Input: part model. Units: mm. Frame: model coordinates. Face numbers are marked on the shaded views. A direction names the side the tool comes from. Round coordinates to 2 decimals unless told otherwise and drop trailing zeros. Loops run counter-clockwise (first coordinate to the right, second up) from the corner with the lowest first, then second, coordinate; pieces in that order, holes last.
1) Ray query, line 1 along X through (y, z) = (8.75, -10); line 2 along Z through (x, y) = (130, 3.25); line 3 along Z through (x, y) = (169, 13.25). Return the intervals inside material, ascending.
2) First-contact query: pin 1 (1.2 mm diameter, centred on x = 75, z = -10, fed in from +Y); pin 2 (1 mm diameter, centred on x = 178, z = 10.5, fed in from -Y); pin 3 (12 mm diameter, centred on x = 121, y = 10.5, fed in from +Z); pin 4 (1.5 mm diameter, centred on y = 9, z = 55.5, fed in from -X). Flat tips, straight axial feed; report the tip coordinate or a pass-through.
3) Access query for the marked faces 1 and 2. Directions: +Z, -Z, +X, -X, +Y, -Y. A direction counts if a zero-diameter tool reaches every point of the face in a straight line with its end or side. Return the directions, or none.
4) Section A-A, the plane z = -114. Return loops of the section in (x, y).
5) Draft query along X for the marked faces 3, 4, 5 and 6. Return one class per face: pulls with the +X half, pulls with the -X half, needs draft (parallel to the pull), parting line crosses it, or undercut.
6) Section B-B, the plane x = 151.5. Return loops of the section in (y, z).
from build123d import *

# Parameters (mm, degrees)
CORNERBOSS_EXTRUDE1_DEPTH               = 20
SHELL1_T                                = -3
PUTBACKPARTOFSHELLBOSS_EXTRUDE1_DEPTH   = 17
TABHOLECUTSSKETCH1_R                    = 1
TABHOLECUTS_EXTRUDE3_DEPTH              = 267.480732183
PADSKETCH2_R                            = 12
PADSKETCH2_R_2                          = 5
PADBOSS_EXTRUDE2_DEPTH                  = 10
STEPPERRODHOLESKETCH3_R                 = 5.1
STEPPERRODHOLESKETCH3_R_2               = 1.5
STEPPERRODHOLECUT_EXTRUDE1_DEPTH        = 267.046951918
THREADEDNUTMOUNTHOLESSKETCH4_R          = 1
THREADEDNUTMOUNTHOLESCUT_EXTRUDE2_DEPTH = 10
TLPEGHOLESKETCH1_W                      = 10
TLPEGHOLESKETCH1_H                      = 14
TLPEGHOLECUT_EXTRUDE1_DEPTH             = 3
BOTTOMPEGSKETCH2_W                      = 9.8
BOTTOMPEGSKETCH2_H                      = 13.9
BOTTOMPEGBOSS_EXTRUDE1_DEPTH            = 3.1
BOTTOMPEGCAPSKETCH3_W                   = 16
BOTTOMPEGCAPSKETCH3_H                   = 17
BOTTOMPEGCAPBOSS_EXTRUDE2_DEPTH         = 3


with BuildPart() as part:
    # CornerSketch1 → CornerBoss-Extrude1 (new body)
    with BuildSketch(Plane(origin=(0, 0, 0), x_dir=(1, 0, 0), z_dir=(0, 1, 0))):
        with BuildLine():
            Line((210, -50), (120, -50))
            Line((120, -50), (120, 0))
            Line((120, 0), (0, 0))
            Line((0, 0), (0, 100))
            Line((0, 100), (176, 100))
            Line((176, 100), (176, 145.825))
            ThreePointArc((176, 145.825), (193, 162.825), (210, 145.825))
            Line((210, 145.825), (210, -50))
        make_face()
    extrude(amount=CORNERBOSS_EXTRUDE1_DEPTH)

    # Shell1
    shell1_openings = [part.faces().sort_by_distance(p)[0] for p in [
        (121.249517572, 0, -43.561989295),
    ]]
    offset(amount=SHELL1_T, openings=shell1_openings, kind=Kind.INTERSECTION)

    # PutBackPartOfShellSketch1 → PutBackPartOfShellBoss-Extrude1 (add)
    with BuildSketch(Plane.XZ.offset(-17)):
        Polygon((3, -3), (123, -3), (123, 47), (143, 47), (143, -23), (3, -23), align=None)
    extrude(amount=PUTBACKPARTOFSHELLBOSS_EXTRUDE1_DEPTH)

    # TabHoleCutsSketch1 → TabHoleCuts-Extrude3 (cut, through all)
    with BuildSketch(Plane.XZ):
        with Locations(Location((130, 30, 0), (0, 0, 270))):
            Circle(TABHOLECUTSSKETCH1_R)
        with Locations(Location((130, -10, 0), (0, 0, 270))):
            Circle(TABHOLECUTSSKETCH1_R)
        with Locations(Location((75, -10, 0), (0, 0, 270))):
            Circle(TABHOLECUTSSKETCH1_R)
        with Locations(Location((20, -10, 0), (0, 0, 270))):
            Circle(TABHOLECUTSSKETCH1_R)
    extrude(amount=-TABHOLECUTS_EXTRUDE3_DEPTH, mode=Mode.SUBTRACT)

    # PadSketch2 → PadBoss-Extrude2 (add)
    with BuildSketch(Plane.XZ.offset(-17)):
        with Locations(Location((193, -145.825, 0), (0, 0, 90))):
            Circle(PADSKETCH2_R)
        with Locations(Location((169, -83, 0), (0, 0, 90))):
            Circle(PADSKETCH2_R_2)
    extrude(amount=PADBOSS_EXTRUDE2_DEPTH)

    # StepperRodHoleSketch3 → StepperRodHoleCut-Extrude1 (cut, through all)
    with BuildSketch(Plane.XZ.offset(-7)):
        with Locations(Location((193, -145.825, 0), (0, 0, 270))):
            Circle(STEPPERRODHOLESKETCH3_R)
        with Locations(Location((169, -83, 0), (0, 0, 270))):
            Circle(STEPPERRODHOLESKETCH3_R_2)
    extrude(amount=-STEPPERRODHOLECUT_EXTRUDE1_DEPTH, mode=Mode.SUBTRACT)

    # ThreadedNutMountHolesSketch4 → ThreadedNutMountHolesCut-Extrude2 (cut)
    with BuildSketch(Plane(origin=(0, 7, 0), x_dir=(-1, 0, 0), z_dir=(0, -1, 0))):
        with Locations(Location((-193, 153.825, 0), (0, 0, 90))):
            Circle(THREADEDNUTMOUNTHOLESSKETCH4_R)
        with Locations(Location((-185, 145.825, 0), (0, 0, 90))):
            Circle(THREADEDNUTMOUNTHOLESSKETCH4_R)
        with Locations(Location((-201, 145.825, 0), (0, 0, 90))):
            Circle(THREADEDNUTMOUNTHOLESSKETCH4_R)
        with Locations(Location((-193, 137.825, 0), (0, 0, 90))):
            Circle(THREADEDNUTMOUNTHOLESSKETCH4_R)
    extrude(amount=-THREADEDNUTMOUNTHOLESCUT_EXTRUDE2_DEPTH, mode=Mode.SUBTRACT)

    # TLPegHoleSketch1 → TLPegHoleCut-Extrude1 (cut)
    with BuildSketch(Plane.ZY):
        with Locations((-85, 7)):
            Rectangle(TLPEGHOLESKETCH1_W, TLPEGHOLESKETCH1_H)
    extrude(amount=-TLPEGHOLECUT_EXTRUDE1_DEPTH, mode=Mode.SUBTRACT)

    # BottomPegSketch2 → BottomPegBoss-Extrude1 (add)
    with BuildSketch(Plane.XY.offset(50)):
        with Locations((195, 6.95)):
            Rectangle(BOTTOMPEGSKETCH2_W, BOTTOMPEGSKETCH2_H)
    extrude(amount=BOTTOMPEGBOSS_EXTRUDE1_DEPTH)

    # BottomPegCapSketch3 → BottomPegCapBoss-Extrude2 (add)
    with BuildSketch(Plane.XY.offset(53.1)):
        with Locations((195.1, 8.5)):
            Rectangle(BOTTOMPEGCAPSKETCH3_W, BOTTOMPEGCAPSKETCH3_H)
    extrude(amount=BOTTOMPEGCAPBOSS_EXTRUDE2_DEPTH)

    # OverlapChamfer1
    # the kernel refuses this chamfer: 20 mm, written as the material it takes off along each edge
    with BuildSketch(Plane(origin=(120, 20, 50), x_dir=(-0.027495876610586317, -0.9996219169112968, 0), z_dir=(0, 0, -1))) as overlapchamfer1_piece_1:
        with BuildLine():
            Line((20.573463904, 0), (-1.130943098, -20.54235587))
            Line((-1.130943098, -20.54235587), (-1.530791864, -20.53135752))
            ThreePointArc((-1.530791864, -20.53135752), (-0.682584541, -10.267956593), (-0.399848767, 0.010998351))
            Line((-0.399848767, 0.010998351), (0.010998351, 0.399848767))
            ThreePointArc((0.010998351, 0.399848767), (10.289953294, 0.117112992), (20.584462254, 0.399848767))
            Line((20.584462254, 0.399848767), (20.573463904, 0))
        make_face()
    extrude(amount=50, mode=Mode.SUBTRACT)
    with BuildSketch(Plane(origin=(120, 20, 0), x_dir=(0, -0.9996219169112968, 0.027495876610586372), z_dir=(-1, 0, 0))) as overlapchamfer1_piece_2:
        with BuildLine():
            Line((20.573463904, 0), (-1.130943098, -20.54235587))
            Line((-1.130943098, -20.54235587), (-1.530791864, -20.53135752))
            ThreePointArc((-1.530791864, -20.53135752), (-0.682584541, -10.267956593), (-0.399848767, 0.010998351))
            Line((-0.399848767, 0.010998351), (0.010998351, 0.399848767))
            ThreePointArc((0.010998351, 0.399848767), (10.289953294, 0.117112992), (20.584462254, 0.399848767))
            Line((20.584462254, 0.399848767), (20.573463904, 0))
        make_face()
    extrude(amount=120, mode=Mode.SUBTRACT)
    with BuildSketch(Plane(origin=(120, 20, 50), x_dir=(-0.027495876610586317, -0.9996219169112968, 0), z_dir=(0, 0, -1))) as overlapchamfer1_piece_3a_section:
        with BuildLine():
            Line((20.573463904, 0), (-1.130943098, -20.54235587))
            Line((-1.130943098, -20.54235587), (-1.530791864, -20.53135752))
            ThreePointArc((-1.530791864, -20.53135752), (-0.682584541, -10.267956593), (-0.399848767, 0.010998351))
            Line((-0.399848767, 0.010998351), (0.010998351, 0.399848767))
            ThreePointArc((0.010998351, 0.399848767), (10.289953294, 0.117112992), (20.584462254, 0.399848767))
            Line((20.584462254, 0.399848767), (20.573463904, 0))
        make_face()
    overlapchamfer1_piece_3a = extrude(amount=101.433659759, mode=Mode.PRIVATE)
    overlapchamfer1_piece_3a = split(overlapchamfer1_piece_3a, bisect_by=Plane(origin=(126.595872536, 13.404127464, 0), z_dir=(0, 0, -1)), keep=Keep.TOP, mode=Mode.PRIVATE)
    with BuildSketch(Plane(origin=(171.433659759, 20, 0), x_dir=(0, -0.9996219169112968, 0.027495876610586372), z_dir=(-1, 0, 0))) as overlapchamfer1_piece_3b_section:
        with BuildLine():
            Line((20.573463904, 0), (-1.130943098, -20.54235587))
            Line((-1.130943098, -20.54235587), (-1.530791864, -20.53135752))
            ThreePointArc((-1.530791864, -20.53135752), (-0.682584541, -10.267956593), (-0.399848767, 0.010998351))
            Line((-0.399848767, 0.010998351), (0.010998351, 0.399848767))
            ThreePointArc((0.010998351, 0.399848767), (10.289953294, 0.117112992), (20.584462254, 0.399848767))
            Line((20.584462254, 0.399848767), (20.573463904, 0))
        make_face()
    overlapchamfer1_piece_3b = extrude(amount=171.433659759, mode=Mode.PRIVATE)
    overlapchamfer1_piece_3b = split(overlapchamfer1_piece_3b, bisect_by=Plane(origin=(120, 13.404127464, -6.595872536), z_dir=(1, 0, 0)), keep=Keep.TOP, mode=Mode.PRIVATE)
    overlapchamfer1_piece_3 = overlapchamfer1_piece_3a & overlapchamfer1_piece_3b
    add(overlapchamfer1_piece_3, mode=Mode.SUBTRACT)


solid = part.part
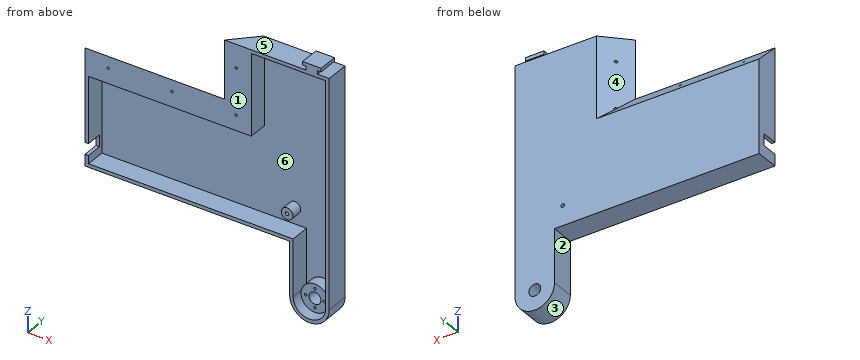
Final values:
1. line 1: x = 0 to 19, 21 to 74, 76 to 129, 131 to 143, 207 to 210
1. line 2: z = -100 to -97, -23 to -11, -9 to 29, 31 to 50
1. line 3: z = -100 to -97, -88 to -84.5, -81.5 to -78, 47 to 50
2. pin 1: passes through
2. pin 2: stops at y = 17
2. pin 3: stops at z = -4.5
2. pin 4: stops at x = 187.1
3. face 1: +Z, -Z, +X, -X, -Y
3. face 2: -Z, -X, +Y, -Y
4. outline: (176, 0) - (179, 0) - (179, 17) - (207, 17) - (207, 0) - (210, 0) - (210, 20) - (176, 20) - close
5. face 3: parting line crosses it
5. face 4: pulls with the -X half
5. face 5: needs draft
5. face 6: undercut
6. outline: (0, -100) - (20, -100) - (20, 50) - (0, 50) - (0, 47) - (17, 47) - (17, -97) - (0, -97) - close
